Drawing for the job (mm, zero at the part's lowest x, y, z). A direction names the side the tool comes from. Coordinates: 2 decimals unless noted, no trailing zeros. Write each loop counter-clockwise with the first axis right and the second up, starting at its lowest first coordinate (ties: lowest second). Pieces come first, ordered by that corner, then holes. Notation, with made-up numbers: M 52.25,56 L 66.25,56 A12 cw 66.25,70 Z; hole C 12.5,74 d9. An arc over 180 degrees is marked long. Put each result on its own line as item: value. Start each with the question number.
Q1. Which spindle directions (+Z, -Z, +X, -X, +Y, -Y) get a long thin tool onto all of the face, cutting with end or side? Do the marked faces 1 and 2. Say none if no direction does.
Q2. Cut at C-C (y = 2.3). Write the cut outline in (x, z).
Q3. Cut at D-D (z = 22). Write the cut outline in (x, y), then the cut area to 3 significant figures.
Q4. Pull direction X, two halves, no side cores. Call the marked faces 3, 4 and 5: pulls with the +X half, pulls with the -X half, needs draft (parallel to the pull), parting line crosses it, or undercut.
Q5. Cut at A-A (z = 12.65). Write the cut outline in (x, y).
Q6. Drill centre lines: line 1 along X through (y, z) = (2, 12.65); line 2 along Z through (x, y) = (10.5, 1.8); line 3 along X through (y, z) = (3.25, 17.5). Where is each one in solid material? Low to high.
Q7. Drop flat-ended pins along their axis: pin 1 (4 mm diameter, centred on x = 15.5, z = 11, fed in from +Y); pin 2 (1 mm diameter, centred on y = 4, z = 7.5, fed in from +X); pin 3 (0.6 mm diameter, centred on y = 4, z = 18, fed in from +X); pin 4 (1.5 mm diameter, centred on y = 4, z = 15.5, fed in from +X). Give the stop position or say it passes through.
Q8. Cut at B-B (x = 12.65). Write the cut outline in (y, z), then the cut area to 4 significant figures.
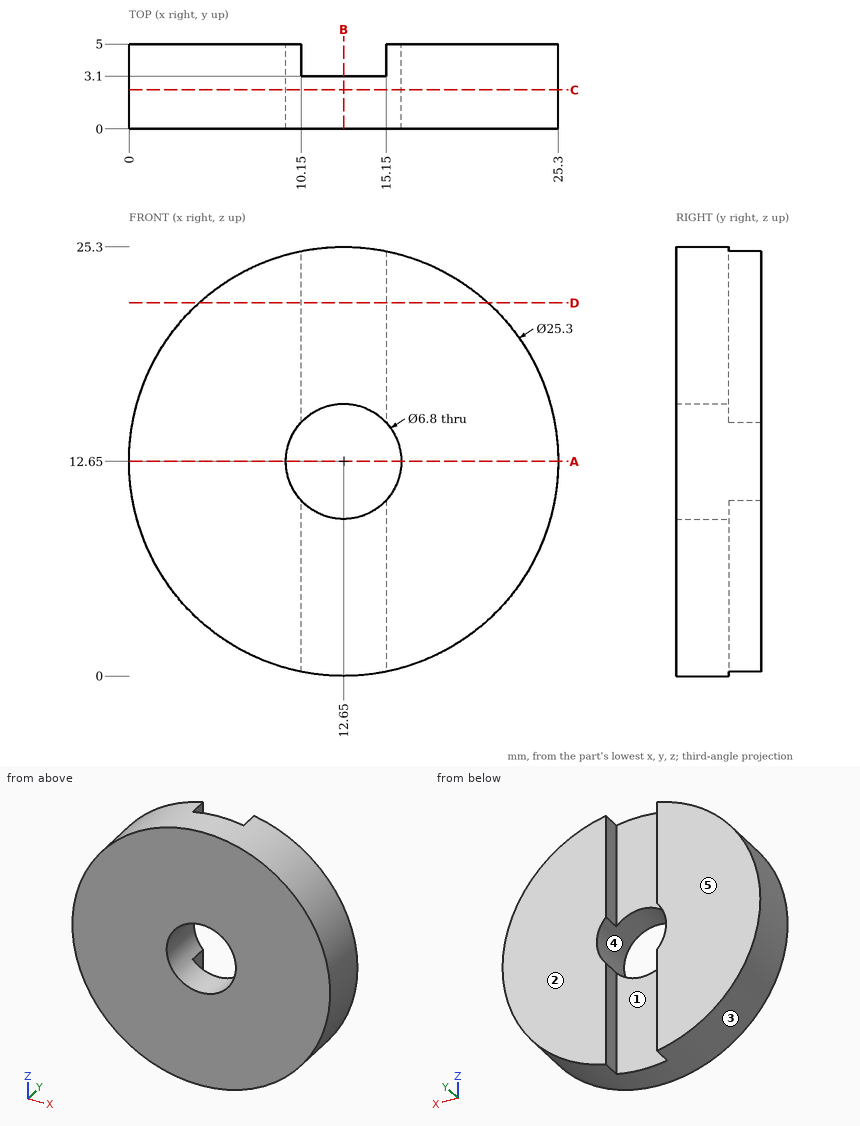
Computed values:
1. face 1: +Z, -Z, +Y
1. face 2: +Z, -Z, +X, -X, +Y
2. outline: C 12.65,12.65 d25.3; hole C 12.65,12.65 d6.8
3. outline: M 4.13,0 L 21.17,0 L 21.17,5 L 15.15,5 L 15.15,3.1 L 10.15,3.1 L 10.15,5 L 4.13,5 Z
3. area: 75.7 mm2
4. face 3: parting line crosses it
4. face 4: undercut
4. face 5: needs draft
5. outline: M 0,0 L 9.25,0 L 9.25,5 L 0,5 Z; M 16.05,0 L 25.3,0 L 25.3,5 L 16.05,5 Z
6. line 1: 0 to 9.25, 16.05 to 25.3
6. line 2: 0.18 to 10.02, 15.28 to 25.12
6. line 3: 0.97 to 10.15, 15.15 to 24.33
7. pin 1: y = 5
7. pin 2: x = 24.41
7. pin 3: x = 24.25
7. pin 4: x = 25.12
8. outline: M 0,0 L 3.1,0 L 3.1,9.25 L 0,9.25 Z; M 0,16.05 L 3.1,16.05 L 3.1,25.3 L 0,25.3 Z
8. area: 57.35 mm2
